Verification items for this drawing (mm, ordinates from the low corner). A direction names the side the tool comes from. Coordinates: 2 decimals unless noted, no trailing zeros. Loops run counter-clockwise (first coordinate to the right, second up) from the corner with the lowest first, then second, coordinate; pieces in that order, holes last. Notation, with made-up numbers: M 45,54.5 L 77,54.5 A26 ccw 77,84.5 Z; hole C -18.5,46.25 d10. An arc over 180 degrees is marked long. Use CSV: the item, a comma, the result in double quotes.
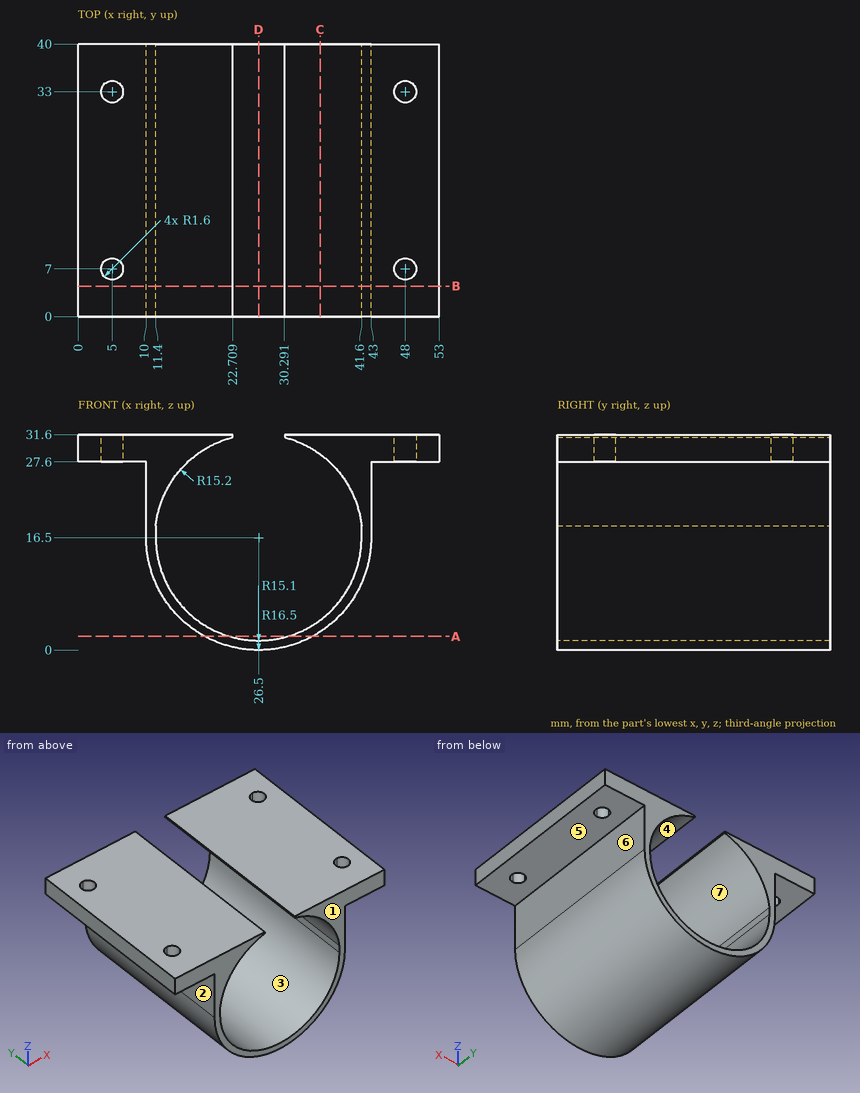
1. Release check for a two-part mould opening along Z. For the marked faces 4, 5, 6 and 7 record: +Z half, -Z half, draft (parallel to the pull), parting line (faces both ways), or undercut.
The answers:
face 4,"undercut"
face 5,"-Z half"
face 6,"draft"
face 7,"undercut"
2. Gauge pin test, flat ends, axial feed: P1, Ø4, axis at y = 13, z = 9.5, coming from the -X side; P2, Ø1.9, axis at y = 15, z = 17.5, coming from the -X side; P3, Ø10, axis at x = 20.5, y = 7, coming from the -Z side. Record the tip position at first contact, or that the pin passes through.
The answers:
P1,"x = 10.78"
P2,"x = 10"
P3,"z = 0.03"
3. Section check D-D, the plane x = 26.5. Record the cut outline in (y, z).
The answers:
outline,"M 0,0 L 40,0 L 40,1.4 L 0,1.4 Z"
4. Set-up check for the marked faces 1, 2 and 3: record each of +Z, -Z, +X, -X, +Y, -Y from which the full face is reachable in a straight line by a thin tool's end or side.
The answers:
face 1,"+Z, -Z, +X, -X, -Y"
face 2,"-Z, -X, +Y, -Y"
face 3,"+Y, -Y"
5. Section check A-A, the plane z = 2. Record the cut outline in (x, y).
The answers:
outline,"M 18.63,0 L 22.29,0 L 22.29,40 L 18.63,40 Z; M 30.71,0 L 34.37,0 L 34.37,40 L 30.71,40 Z"
6. Thickness scan on line 1 (X direction, y = 20, z = 17); line 2 (Z direction, x = 9, y = 19); line 3 (X direction, y = 36.5, z = 8.5). Record the ranges inside material, lowest first. Write a range as [from, to].
The answers:
line 1,"[10, 11.4], [41.6, 43]"
line 2,"[27.6, 31.6]"
line 3,"[12.07, 13.69], [39.31, 40.93]"
7. Section check B-B, the plane y = 4.5. Record the cut outline in (x, z).
The answers:
outline,"M 0,27.6 L 10,27.6 L 10,16.5 A16.5 ccw 43,16.5 L 43,27.6 L 53,27.6 L 53,31.6 L 30.29,31.6 L 30.29,31.22 A15.2 cw 41.6,18.24 L 41.6,16.5 A15.1 cw 11.4,16.5 L 11.4,18.24 A15.2 cw 22.71,31.22 L 22.71,31.6 L 0,31.6 Z"
8. Section check C-C, the plane x = 35.5. Record the cut outline in (y, z) (1 decimal), plus the area to 3 significant figures.
The answers:
outline,"M 0,2.7 L 40,2.7 L 40,4.4 L 0,4.4 Z; M 0,28.7 L 40,28.7 L 40,31.6 L 0,31.6 Z"
area,"182 mm^2"
